Input: part model. Units: mm. Frame: model coordinates. A direction names the side the tool comes from. Coordinates: 2 decimals unless noted, no trailing zeros. Order: outer loops, then holes, each group sorted by start corner. A loop starts at its lowest first (then second) coordinate and runs counter-clockwise, first axis right, second up. Notation, with made-up numbers: M -14,24 L -5,24 A18 ccw -5,33 Z; hole C -33.75,-15 d1. An arc over 180 degrees is marked long. Answer in a Markdown table with one row per item.
from build123d import *

# Parameters (mm, degrees)
BOSS_EXTRUDE1_DEPTH  = 25
FILLET1_R            = 4.5
FILLET2_R            = 9
M6_CLEARANCE_HOLE1_D = 6.6
M5_CLEARANCE_HOLE1_D = 5.5
CHAMFER1_SIZE        = 2


with BuildPart() as part:
    # Sketch1 → Boss-Extrude1 (new body, symmetric)
    with BuildSketch(Plane(origin=(0, 0, 0), x_dir=(0, 0, -1), z_dir=(1, 0, 0))):
        Polygon((0, 0), (-40, 0), (-40, 4.5), (-4.5, 4.5), (-4.5, 146), (0, 146), align=None)
    extrude(amount=BOSS_EXTRUDE1_DEPTH, both=True)

    # Fillet1
    fillet1_edges = [part.edges().sort_by_distance(p)[0] for p in [
        (0, 4.5, 4.5),
    ]]
    fillet(fillet1_edges, radius=FILLET1_R)

    # Fillet2
    fillet2_edges = [part.edges().sort_by_distance(p)[0] for p in [
        (0, 0, 0),
    ]]
    fillet(fillet2_edges, radius=FILLET2_R)

    # M6 Clearance Hole1 (through all)
    with Locations(Plane(origin=(0, 4.5, 0), x_dir=(-1, 0, 0), z_dir=(0, 1, 0))):
        with Locations((15, 25), (-15, 25)):
            Hole(M6_CLEARANCE_HOLE1_D / 2)

    # M5 Clearance Hole1 (through all)
    with Locations(Plane(origin=(0, 0, 0), x_dir=(-1, 0, 0), z_dir=(0, 0, -1))):
        with Locations((18, 132.7), (0, 132.7), (0, 95.3), (18, 95.3)):
            Hole(M5_CLEARANCE_HOLE1_D / 2)

    # Chamfer1
    chamfer1_edges = [part.edges().sort_by_distance(p)[0] for p in [
        (25, 2.25, 40),
        (25, 146, 2.25),
        (-25, 146, 2.25),
        (-25, 2.25, 40),
    ]]
    chamfer(chamfer1_edges, length=CHAMFER1_SIZE)


solid = part.part
1) Material intervals for probe 1 along X at (y, z) = (132.7, 2.05); probe 2 along Z at (x, y) = (-2.5, 125), sorted ascending.
Resolved:
| item | result |
|---|---|
| probe 1 | x = -25 to -20.75, -15.25 to -2.75, 2.75 to 25 |
| probe 2 | z = 0 to 4.5 |
2) Cut plane C-C, the plane y = 132.7. Output: boundary loops of the cut face in (x, z).
Resolved:
| item | result |
|---|---|
| outline | M -25,0 L -20.75,0 L -20.75,4.5 L -25,4.5 Z; M -15.25,0 L -2.75,0 L -2.75,4.5 L -15.25,4.5 Z; M 2.75,0 L 25,0 L 25,4.5 L 2.75,4.5 Z |
3) Mould query, pull axis Z, two halves, no side actions, for faces 1 (the face through (0, 4.5, 25)), 2 (the face through (0.35, 2.566, 2.706)), 3 (the face through (-0.35, 5.853, 5.783)), 4 (the face through (14.28, 2.22, 21.78)). Classes: +Z half, -Z half, draft (parallel to the pull), parting line (faces both ways), or undercut.
Resolved:
| item | result |
|---|---|
| face 1 | draft |
| face 2 | -Z half |
| face 3 | +Z half |
| face 4 | undercut |
4) Cut plane D-D, the plane x = 0. Output: boundary loops of the cut face in (y, z).
Resolved:
| item | result |
|---|---|
| outline | M 0,9 A9 ccw 9,0 L 92.55,0 L 92.55,4.5 L 9,4.5 A4.5 cw 4.5,9 L 4.5,40 L 0,40 Z; M 98.05,0 L 129.95,0 L 129.95,4.5 L 98.05,4.5 Z; M 135.45,0 L 146,0 L 146,4.5 L 135.45,4.5 Z |
5) Reachability of faces 5 (the face through (0, 77, 4.5)), 6 (the face through (-18.596, 130.015, 2.281)) from +Z, -Z, +X, -X, +Y, -Y: full face, straight path, thin tool, end or side. Return the list, or none.
Resolved:
| item | result |
|---|---|
| face 5 | +Z, +X, -X, +Y |
| face 6 | +Z, -Z |
6) Contact query for flat-ended pins moving along their axis: pin 1 (4.5 mm diameter, centred on x = 0, y = 95.3, fed in from -Z); pin 2 (15.5 mm diameter, centred on x = 7.5, z = 32, fed in from +Y); pin 3 (9 mm diameter, centred on x = -18, y = 132.7, fed in from +Z). Output: stop coordinate, or through.
Resolved:
| item | result |
|---|---|
| pin 1 | passes through |
| pin 2 | stops at y = 4.5 |
| pin 3 | stops at z = 4.5 |
7) Cut plane A-A, the plane x = 15. Output: boundary loops of the cut face in (y, z), and give its area (3 significant figures).
Resolved:
| item | result |
|---|---|
| outline | M 0,9 A9 ccw 9,0 L 146,0 L 146,4.5 L 9,4.5 A4.5 cw 4.5,9 L 4.5,21.7 L 0,21.7 Z; M 0,28.3 L 4.5,28.3 L 4.5,40 L 0,40 Z |
| area | 774 mm2 |
8) Cut plane B-B, the plane z = 25. Output: boundary loops of the cut face in (x, y).
Resolved:
| item | result |
|---|---|
| outline | M -25,0 L -18.3,0 L -18.3,4.5 L -25,4.5 Z; M -11.7,0 L 11.7,0 L 11.7,4.5 L -11.7,4.5 Z; M 18.3,0 L 25,0 L 25,4.5 L 18.3,4.5 Z |
